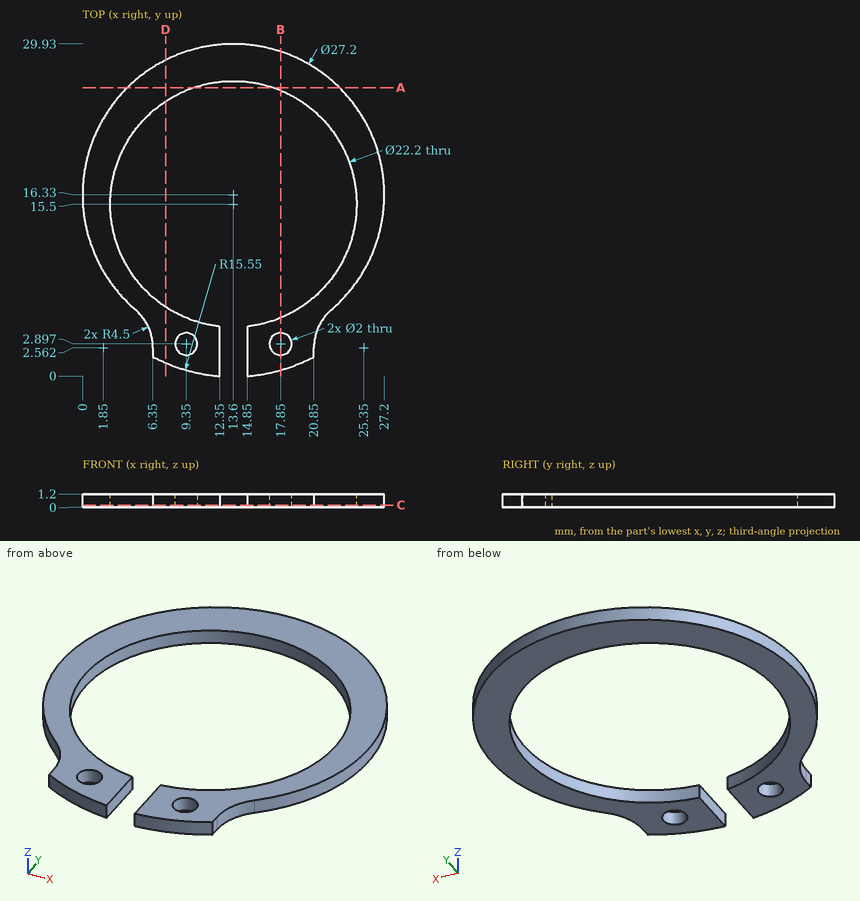
Check sheet for the drawn part. Datum: minimum x, y, z corner. Units: mm. Round coordinates to 2 decimals unless told otherwise and drop trailing zeros. Order: outer loops, then holes, each group sorted by start corner. A loop starts at its lowest first (then second) coordinate and runs counter-clockwise, first axis right, second up. Notation, with made-up numbers: (-25, 14) -> (-1, 14) arc R37 cw to (-1, 52) -> close; hole circle Ø11 at (-31, 30.5). An arc over 180 degrees is marked (long way). Return JSON: item names as keys, results as strings. Group by question number.
Q1. Section check A-A, the plane y = 26. Record the boundary of the cut face in (x, z).
Q2. Material ranges on probe 1 along X at (y, z) = (3.75, 0.9); probe 2 along Y at (x, z) = (17.85, 0.85) (1 decimal); probe 3 along Y at (x, z) = (17.75, 0.45) (1 decimal), recorded low to high. Write a range as from..to.
Q3. Section check C-C, the plane z = 0.2. Count the separate pieces of the cut face and the enclosed holes in it.
Q4. Section check B-B, the plane x = 17.85. Record the boundary of the cut face in (y, z) (1 decimal).
Q5. Section check D-D, the plane x = 7.5. Record the boundary of the cut face in (y, z) (1 decimal).
Q6. Gauge pin test, flat end, axial feed: pin 1 (0.7 mm diameter, centred on y = 2, z = 0.5, fed in from +X). Record the tip position at first contact, or that the pin passes through.
Numbers:
{
 "1": {"outline": "(4.04, 0) -> (10, 0) -> (10, 1.2) -> (4.04, 1.2) -> close; (17.2, 0) -> (23.16, 0) -> (23.16, 1.2) -> (17.2, 1.2) -> close"},
 "2": {"probe 1": "6.19..8.83, 9.87..12.35, 14.85..17.33, 18.37..21.01", "probe 2": "0.5..1.9, 3.9..5.2, 25.8..29.2", "probe 3": "0.5..1.9, 3.9..5.2, 25.8..29.3"},
 "3": {"separate pieces": "1", "enclosed holes": "2"},
 "4": {"outline": "(0.5, 0) -> (1.9, 0) -> (1.9, 1.2) -> (0.5, 1.2) -> close; (3.9, 0) -> (5.2, 0) -> (5.2, 1.2) -> (3.9, 1.2) -> close; (25.8, 0) -> (29.2, 0) -> (29.2, 1.2) -> (25.8, 1.2) -> close"},
 "5": {"outline": "(1.2, 0) -> (6.2, 0) -> (6.2, 1.2) -> (1.2, 1.2) -> close; (24.8, 0) -> (28.5, 0) -> (28.5, 1.2) -> (24.8, 1.2) -> close"},
 "6": {"pin 1": "x = 20.85"}
}
